from build123d import *

# Parameters (mm, degrees)
BOSS_EXTRUDE1_DEPTH = 6
SKETCH2_R           = 1.5
CUT_EXTRUDE1_DEPTH  = 107.235587258


with BuildPart() as part:
    # Sketch1 → Boss-Extrude1 (new body)
    with BuildSketch(Plane(origin=(0, 0, 0), x_dir=(1, 0, 0), z_dir=(0, 1, 0))):
        Polygon((0, 75), (25, 75), (25, 69), (50, 69), (50, 75), (69, 75), (69, 50), (75, 50), (75, 25), (69, 25), (69, 0), (75, 0), (75, -25), (69, -25), (69, -50), (75, -50), (75, -69), (50, -69), (50, -75), (25, -75), (25, -69), (0, -69), (0, -75), (-25, -75), (-25, -69), (-50, -69), (-50, -75), (-69, -75), (-69, -50), (-75, -50), (-75, -25), (-69, -25), (-69, 0), (-75, 0), (-75, 25), (-69, 25), (-69, 50), (-75, 50), (-75, 69), (-50, 69), (-50, 75), (-25, 75), (-25, 69), (0, 69), align=None)
    extrude(amount=BOSS_EXTRUDE1_DEPTH)

    # Sketch2 → Cut-Extrude1 (cut, through all)
    with BuildSketch(Plane(origin=(0, 6, 0), x_dir=(1, 0, 0), z_dir=(0, 1, 0))):
        with Locations(Location((-37.5, 72, 0), (0, 0, 270))):
            Circle(SKETCH2_R)
        with Locations(Location((12.5, 72, 0), (0, 0, 270))):
            Circle(SKETCH2_R)
        with Locations(Location((72, 37.5, 0), (0, 0, 270))):
            Circle(SKETCH2_R)
        with Locations(Location((72, -12.5, 0), (0, 0, 270))):
            Circle(SKETCH2_R)
        with Locations(Location((37.5, -72, 0), (0, 0, 270))):
            Circle(SKETCH2_R)
        with Locations(Location((-12.5, -72, 0), (0, 0, 270))):
            Circle(SKETCH2_R)
        with Locations(Location((-72, -37.5, 0), (0, 0, 270))):
            Circle(SKETCH2_R)
        with Locations(Location((-72, 12.5, 0), (0, 0, 270))):
            Circle(SKETCH2_R)
        with BuildLine():
            Line((-11, 69), (-14, 69))
            Line((-14, 69), (-14, 66.6))
            Line((-14, 66.6), (-15.1, 66.6))
            ThreePointArc((-15.1, 66.6), (-15.270710678, 66.670710678), (-15.2, 66.5))
            Line((-15.2, 66.5), (-15.2, 64.3))
            ThreePointArc((-15.2, 64.3), (-15.270710678, 64.129289322), (-15.1, 64.2))
            Line((-15.1, 64.2), (-14, 64.2))
            Line((-14, 64.2), (-14, 63))
            Line((-14, 63), (-11, 63))
            Line((-11, 63), (-11, 64.2))
            Line((-11, 64.2), (-9.9, 64.2))
            ThreePointArc((-9.9, 64.2), (-9.729289322, 64.129289322), (-9.8, 64.3))
            Line((-9.8, 64.3), (-9.8, 66.5))
            ThreePointArc((-9.8, 66.5), (-9.729289322, 66.670710678), (-9.9, 66.6))
            Line((-9.9, 66.6), (-11, 66.6))
            Line((-11, 66.6), (-11, 69))
        make_face()
        with BuildLine():
            Line((69, 11), (69, 14))
            Line((69, 14), (66.6, 14))
            Line((66.6, 14), (66.6, 15.1))
            ThreePointArc((66.6, 15.1), (66.670710678, 15.270710678), (66.5, 15.2))
            Line((66.5, 15.2), (64.3, 15.2))
            ThreePointArc((64.3, 15.2), (64.129289322, 15.270710678), (64.2, 15.1))
            Line((64.2, 15.1), (64.2, 14))
            Line((64.2, 14), (63, 14))
            Line((63, 14), (63, 11))
            Line((63, 11), (64.2, 11))
            Line((64.2, 11), (64.2, 9.9))
            ThreePointArc((64.2, 9.9), (64.129289322, 9.729289322), (64.3, 9.8))
            Line((64.3, 9.8), (66.5, 9.8))
            ThreePointArc((66.5, 9.8), (66.670710678, 9.729289322), (66.6, 9.9))
            Line((66.6, 9.9), (66.6, 11))
            Line((66.6, 11), (69, 11))
        make_face()
        with BuildLine():
            Line((39, 69), (36, 69))
            Line((36, 69), (36, 66.6))
            Line((36, 66.6), (34.9, 66.6))
            ThreePointArc((34.9, 66.6), (34.729289322, 66.670710678), (34.8, 66.5))
            Line((34.8, 66.5), (34.8, 64.3))
            ThreePointArc((34.8, 64.3), (34.729289322, 64.129289322), (34.9, 64.2))
            Line((34.9, 64.2), (36, 64.2))
            Line((36, 64.2), (36, 63))
            Line((36, 63), (39, 63))
            Line((39, 63), (39, 64.2))
            Line((39, 64.2), (40.1, 64.2))
            ThreePointArc((40.1, 64.2), (40.270710678, 64.129289322), (40.2, 64.3))
            Line((40.2, 64.3), (40.2, 66.5))
            ThreePointArc((40.2, 66.5), (40.270710678, 66.670710678), (40.1, 66.6))
            Line((40.1, 66.6), (39, 66.6))
            Line((39, 66.6), (39, 69))
        make_face()
        with BuildLine():
            Line((69, -39), (69, -36))
            Line((69, -36), (66.6, -36))
            Line((66.6, -36), (66.6, -34.9))
            ThreePointArc((66.6, -34.9), (66.670710678, -34.729289322), (66.5, -34.8))
            Line((66.5, -34.8), (64.3, -34.8))
            ThreePointArc((64.3, -34.8), (64.129289322, -34.729289322), (64.2, -34.9))
            Line((64.2, -34.9), (64.2, -36))
            Line((64.2, -36), (63, -36))
            Line((63, -36), (63, -39))
            Line((63, -39), (64.2, -39))
            Line((64.2, -39), (64.2, -40.1))
            ThreePointArc((64.2, -40.1), (64.129289322, -40.270710678), (64.3, -40.2))
            Line((64.3, -40.2), (66.5, -40.2))
            ThreePointArc((66.5, -40.2), (66.670710678, -40.270710678), (66.6, -40.1))
            Line((66.6, -40.1), (66.6, -39))
            Line((66.6, -39), (69, -39))
        make_face()
        with BuildLine():
            Line((11, -69), (14, -69))
            Line((14, -69), (14, -66.6))
            Line((14, -66.6), (15.1, -66.6))
            ThreePointArc((15.1, -66.6), (15.270710678, -66.670710678), (15.2, -66.5))
            Line((15.2, -66.5), (15.2, -64.3))
            ThreePointArc((15.2, -64.3), (15.270710678, -64.129289322), (15.1, -64.2))
            Line((15.1, -64.2), (14, -64.2))
            Line((14, -64.2), (14, -63))
            Line((14, -63), (11, -63))
            Line((11, -63), (11, -64.2))
            Line((11, -64.2), (9.9, -64.2))
            ThreePointArc((9.9, -64.2), (9.729289322, -64.129289322), (9.8, -64.3))
            Line((9.8, -64.3), (9.8, -66.5))
            ThreePointArc((9.8, -66.5), (9.729289322, -66.670710678), (9.9, -66.6))
            Line((9.9, -66.6), (11, -66.6))
            Line((11, -66.6), (11, -69))
        make_face()
        with BuildLine():
            Line((-39, -69), (-36, -69))
            Line((-36, -69), (-36, -66.6))
            Line((-36, -66.6), (-34.9, -66.6))
            ThreePointArc((-34.9, -66.6), (-34.729289322, -66.670710678), (-34.8, -66.5))
            Line((-34.8, -66.5), (-34.8, -64.3))
            ThreePointArc((-34.8, -64.3), (-34.729289322, -64.129289322), (-34.9, -64.2))
            Line((-34.9, -64.2), (-36, -64.2))
            Line((-36, -64.2), (-36, -63))
            Line((-36, -63), (-39, -63))
            Line((-39, -63), (-39, -64.2))
            Line((-39, -64.2), (-40.1, -64.2))
            ThreePointArc((-40.1, -64.2), (-40.270710678, -64.129289322), (-40.2, -64.3))
            Line((-40.2, -64.3), (-40.2, -66.5))
            ThreePointArc((-40.2, -66.5), (-40.270710678, -66.670710678), (-40.1, -66.6))
            Line((-40.1, -66.6), (-39, -66.6))
            Line((-39, -66.6), (-39, -69))
        make_face()
        with BuildLine():
            Line((-69, 39), (-69, 36))
            Line((-69, 36), (-66.6, 36))
            Line((-66.6, 36), (-66.6, 34.9))
            ThreePointArc((-66.6, 34.9), (-66.670710678, 34.729289322), (-66.5, 34.8))
            Line((-66.5, 34.8), (-64.3, 34.8))
            ThreePointArc((-64.3, 34.8), (-64.129289322, 34.729289322), (-64.2, 34.9))
            Line((-64.2, 34.9), (-64.2, 36))
            Line((-64.2, 36), (-63, 36))
            Line((-63, 36), (-63, 39))
            Line((-63, 39), (-64.2, 39))
            Line((-64.2, 39), (-64.2, 40.1))
            ThreePointArc((-64.2, 40.1), (-64.129289322, 40.270710678), (-64.3, 40.2))
            Line((-64.3, 40.2), (-66.5, 40.2))
            ThreePointArc((-66.5, 40.2), (-66.670710678, 40.270710678), (-66.6, 40.1))
            Line((-66.6, 40.1), (-66.6, 39))
            Line((-66.6, 39), (-69, 39))
        make_face()
        with BuildLine():
            Line((-69, -11), (-69, -14))
            Line((-69, -14), (-66.6, -14))
            Line((-66.6, -14), (-66.6, -15.1))
            ThreePointArc((-66.6, -15.1), (-66.670710678, -15.270710678), (-66.5, -15.2))
            Line((-66.5, -15.2), (-64.3, -15.2))
            ThreePointArc((-64.3, -15.2), (-64.129289322, -15.270710678), (-64.2, -15.1))
            Line((-64.2, -15.1), (-64.2, -14))
            Line((-64.2, -14), (-63, -14))
            Line((-63, -14), (-63, -11))
            Line((-63, -11), (-64.2, -11))
            Line((-64.2, -11), (-64.2, -9.9))
            ThreePointArc((-64.2, -9.9), (-64.129289322, -9.729289322), (-64.3, -9.8))
            Line((-64.3, -9.8), (-66.5, -9.8))
            ThreePointArc((-66.5, -9.8), (-66.670710678, -9.729289322), (-66.6, -9.9))
            Line((-66.6, -9.9), (-66.6, -11))
            Line((-66.6, -11), (-69, -11))
        make_face()
    extrude(amount=-CUT_EXTRUDE1_DEPTH, mode=Mode.SUBTRACT)


solid = part.part
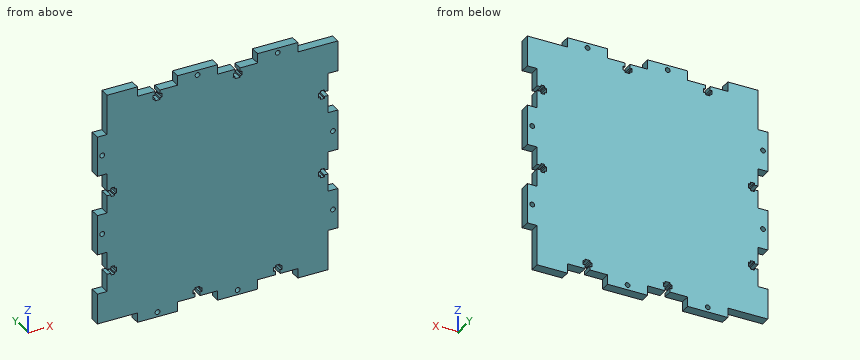
Design review of the part built by this model. Coordinates are the model's own, in mm. Round coordinates to 2 decimals unless told otherwise and drop trailing zeros. Write each loop counter-clockwise with the first axis right and the second up, starting at its lowest first coordinate (ties: lowest second). Pieces come first, ordered by that corner, then holes. Notation, with made-up numbers: (50, 56.5) -> (75, 56.5) arc R28 ccw to (75, 93.5) -> close; hole circle Ø4 at (-21.75, 88). An arc over 180 degrees is marked (long way). One line per item, written item: value. Start each with the question number.
Q1. Add section A-A (z = -61). Give the boundary of the cut face in (x, y), then the cut area to 3 significant figures.
Q2. To check wall thickness, follow probe 1 along Z at (x, y) = (-65.5, 3.2); probe 2 along Z at (x, y) = (-64, 3.55). State the ranges of each line that lie inside material, in increasing order.
Q3. Insertion check: P1, Ø1.8, axis at x = 4, y = 4, coming from the +Z side; P2, Ø0.9, axis at x = 37, y = 4, coming from the -Z side; P3, Ø1.8, axis at y = 4, z = 28, coming from the +X side. Each pin has a flat end and moves straight along its axis. Give the tip position at first contact, or say it passes through.
Q4. Add section B-B (y = 1). State how many separate pieces and enclosed holes the cut face has, then the cut area to 3 significant figures.
Response:
1. outline: (-75, 0) -> (69, 0) -> (69, 6) -> (-75, 6) -> close
1. area: 864 mm^2
2. probe 1: z = -69 to -40.2, -34.8 to 9.8, 15.2 to 75
2. probe 2: z = -69 to -39, -36 to 11, 14 to 75
3. P1: stops at z = 69
3. P2: stops at z = -63
3. P3: stops at x = 69
4. separate pieces: 1
4. enclosed holes: 8
4. area: 20,500 mm^2
